Build history of the part. All positions in model axes, mm. Face numbers are marked on the shaded views. A direction names the side the tool comes from. Give positions to 0.01 mm unless a question says otherwise; leave off trailing zeros. Loops run counter-clockwise (first coordinate to the right, second up) from the corner with the lowest first, then second, coordinate; pieces in that order, holes last. Notation, with made-up numbers: M 46,19 L 75,19 A26 cw 75,50 Z; hole C 10.5,63.5 d4. An arc over 180 degrees is marked long. Put each result on its own line as item: value.
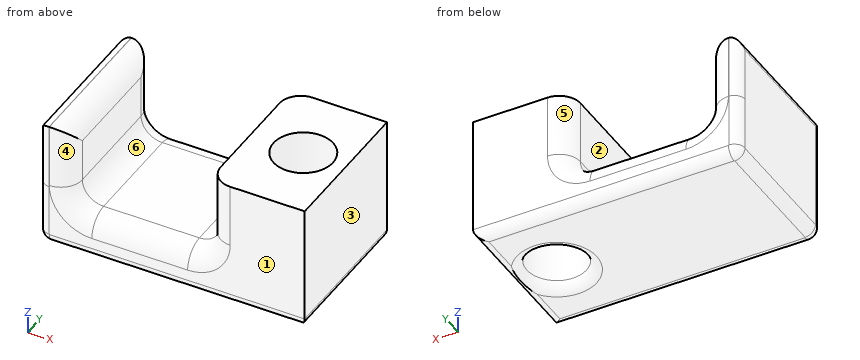
```python
from build123d import *

# Parameters (mm, degrees)
F0_W         = 1.5
F0_H         = 7
F0_W_2       = 6.5
F0_W_3       = 4.5
F0_R         = 1.4
F1_DEPTH     = 2
F2_DEPTH     = 4
F3_F1_R      = 1
F3_F2_R      = 1
F4_T1_DEPTH  = 5.9980686292
F4_T3_DEPTH  = 13.2514489274
F4_T5_DEPTH  = 9.5048292256
F4_T7_DEPTH  = 2.4368940733
F4_T9_DEPTH  = 4.3169803418
F4_T11_DEPTH = 9.509680201
F4_T13_DEPTH = 4.2548401974
F4_T15_DEPTH = 2.4990342177
F4_S19_W     = 0.551502254
F4_S19_H     = 0.5515022539
F4_T20_DEPTH = 0.551502254
F4_S25_W     = 0.551502254
F4_S25_H     = 0.5515022539
F4_T26_DEPTH = 0.551502254


# Not quite as in the source:
# - a fillet or chamfer that OpenCascade refuses, or shapes differently, is made with other operations: its cross-section is extruded or revolved along the edge and cut away or added


with BuildPart() as f1:
    # F0 (on Top) → F1 (new body)
    with BuildSketch(Plane.XY):
        with Locations((-7.4809225276, 0.9873391916)):
            Rectangle(F0_W, F0_H)
        with Locations((-3.4809225276, 0.9873391916)):
            Rectangle(F0_W_2, F0_H)
        with Locations((2.0190774724, 0.9873391916)):
            Rectangle(F0_W_3, F0_H)
        with Locations((2.2690774724, 0.9873391916)):
            Circle(F0_R, mode=Mode.SUBTRACT)
    extrude(amount=-F1_DEPTH)

    # F0 (on Top) → F2 (join)
    with BuildSketch(Plane.XY):
        with Locations((-7.4809225276, 0.9873391916)):
            Rectangle(F0_W, F0_H)
        with Locations((2.0190774724, 0.9873391916)):
            Rectangle(F0_W_3, F0_H)
        with Locations((2.2690774724, 0.9873391916)):
            Circle(F0_R, mode=Mode.SUBTRACT)
    extrude(amount=F2_DEPTH)

    # F3: fillet of radius 1 on 7 edges, made by hand

    # F3_f1
    f3_f1_edges = [f1.edges().sort_by_distance(p)[0] for p in [
        (-0.2309225276, 0.9873391916, 0),
        (-6.7309225276, 0.9873391916, 0),
    ]]
    fillet(f3_f1_edges, radius=F3_F1_R)

    # F3_f2
    f3_f2_edges = [f1.edges().sort_by_distance(p)[0] for p in [
        (-3.4809225276, 4.4873391916, 0),
        (-3.4809225276, -2.5126608084, 0),
        (-6.7309225276, -2.5126608084, 2.5),
        (-6.7309225276, 4.4873391916, 2.5),
        (-6.7309225276, 0.9873391916, 4),
        (-6.4380293088, 4.4873391916, 0.2928932188),
        (-6.4380293088, -2.5126608084, 0.2928932188),
        (-0.5238157464, -2.5126608084, 0.2928932188),
        (-0.5238157464, 4.4873391916, 0.2928932188),
    ]]
    fillet(f3_f2_edges, radius=F3_F2_R)

    # F4: fillet of radius 0.5 on 8 edges, made by hand

    # F4_s2 → F4_t1 (cut)
    with BuildSketch(Plane.XZ.offset(-3.9863735062)):
        with BuildLine():
            ThreePointArc((-8.2313225276, -1.4990343146), (-8.0844759182, -1.8535533906), (-7.7299568422, -2.0004))
            Line((-7.7299568422, -2.0004), (-7.7299568422, -2.0505365685))
            ThreePointArc((-7.7299568422, -2.0505365685), (-7.9804396849, -2.0501365685), (-8.2309225276, -2.0501365685))
            Line((-8.2309225276, -2.0501365685), (-8.2810590962, -2))
            ThreePointArc((-8.2810590962, -2), (-8.2810590962, -1.7495171573), (-8.2814590962, -1.4990343146))
            Line((-8.2814590962, -1.4990343146), (-8.2313225276, -1.4990343146))
        make_face()
    extrude(amount=F4_T1_DEPTH, mode=Mode.SUBTRACT)

    # F4_s4 → F4_t3 (cut)
    with BuildSketch(Plane.YZ.offset(-7.7299568422)):
        with BuildLine():
            ThreePointArc((-2.011695123, -2.0004), (-2.366214199, -1.8535533906), (-2.5130608084, -1.4990343146))
            Line((-2.5130608084, -1.4990343146), (-2.563197377, -1.4990343146))
            ThreePointArc((-2.563197377, -1.4990343146), (-2.562797377, -1.7495171573), (-2.562797377, -2))
            Line((-2.562797377, -2), (-2.5126608084, -2.0501365685))
            ThreePointArc((-2.5126608084, -2.0501365685), (-2.2621779657, -2.0501365685), (-2.011695123, -2.0505365685))
            Line((-2.011695123, -2.0505365685), (-2.011695123, -2.0004))
        make_face()
        with BuildLine():
            ThreePointArc((4.4877391916, -1.4990343146), (4.3408925822, -1.8535533906), (3.9863735062, -2.0004))
            Line((3.9863735062, -2.0004), (3.9863735062, -2.0505365685))
            ThreePointArc((3.9863735062, -2.0505365685), (4.2368563489, -2.0501365685), (4.4873391916, -2.0501365685))
            Line((4.4873391916, -2.0501365685), (4.5374757601, -2))
            ThreePointArc((4.5374757601, -2), (4.5374757601, -1.7495171573), (4.5378757601, -1.4990343146))
            Line((4.5378757601, -1.4990343146), (4.4877391916, -1.4990343146))
        make_face()
    extrude(amount=F4_T3_DEPTH, mode=Mode.SUBTRACT)

    # F4_s6 → F4_t5 (cut)
    with BuildSketch(Plane.XZ.offset(-5.7397538044)):
        with BuildLine():
            ThreePointArc((3.768111787, -2.0004), (4.122630863, -1.8535533906), (4.2694774724, -1.4990343146))
            Line((4.2694774724, -1.4990343146), (4.3196140409, -1.4990343146))
            ThreePointArc((4.3196140409, -1.4990343146), (4.3192140409, -1.7495171573), (4.3192140409, -2))
            Line((4.3192140409, -2), (4.2690774724, -2.0501365685))
            ThreePointArc((4.2690774724, -2.0501365685), (4.0185946297, -2.0501365685), (3.768111787, -2.0505365685))
            Line((3.768111787, -2.0505365685), (3.768111787, -2.0004))
        make_face()
    extrude(amount=F4_T5_DEPTH, mode=Mode.SUBTRACT)

    # F4_s8 → F4_t7 (cut)
    with BuildSketch(Plane.XY.offset(-1.4990343146)):
        with BuildLine():
            ThreePointArc((-8.2313225276, -2.011695123), (-8.0844759182, -2.366214199), (-7.7299568422, -2.5130608084))
            Line((-7.7299568422, -2.5130608084), (-7.7299568422, -2.563197377))
            ThreePointArc((-7.7299568422, -2.563197377), (-7.9804396849, -2.562797377), (-8.2309225276, -2.562797377))
            Line((-8.2309225276, -2.562797377), (-8.2810590962, -2.5126608084))
            ThreePointArc((-8.2810590962, -2.5126608084), (-8.2810590962, -2.2621779657), (-8.2814590962, -2.011695123))
            Line((-8.2814590962, -2.011695123), (-8.2313225276, -2.011695123))
        make_face()
    extrude(amount=F4_T7_DEPTH, mode=Mode.SUBTRACT)

    # F4_s10 → F4_t9 (cut)
    with BuildSketch(Plane.XY.offset(0.9378597587)):
        with BuildLine():
            ThreePointArc((-8.2313225276, -2.0116941886), (-8.0841327357, -2.3665561153), (-7.7289866453, -2.5130589353))
            Line((-7.7289866453, -2.5130589353), (-7.7288896256, -2.56319541))
            ThreePointArc((-7.7288896256, -2.56319541), (-7.7309225276, -2.562797377), (-8.2309225276, -2.562797377))
            Line((-8.2309225276, -2.562797377), (-8.2810590962, -2.5126608084))
            ThreePointArc((-8.2810590962, -2.5126608084), (-8.2810590962, -2.2621774985), (-8.2814590962, -2.0116941886))
            Line((-8.2814590962, -2.0116941886), (-8.2313225276, -2.0116941886))
        make_face()
    extrude(amount=F4_T9_DEPTH, mode=Mode.SUBTRACT)

    # F4_s12 → F4_t11 (cut)
    with BuildSketch(Plane.XZ.offset(-5.7421792921)):
        with BuildLine():
            ThreePointArc((-7.7289866453, 4.0003981269), (-8.0841327357, 3.8538953069), (-8.2313225276, 3.4990333802))
            Line((-8.2313225276, 3.4990333802), (-8.2814590962, 3.4990333802))
            ThreePointArc((-8.2814590962, 3.4990333802), (-8.2810590962, 3.7495166901), (-8.2810590962, 4))
            Line((-8.2810590962, 4), (-8.2309225276, 4.0501365685))
            ThreePointArc((-8.2309225276, 4.0501365685), (-7.7309225276, 4.0501365685), (-7.7288896256, 4.0505346016))
            Line((-7.7288896256, 4.0505346016), (-7.7289866453, 4.0003981269))
        make_face()
    extrude(amount=F4_T11_DEPTH, mode=Mode.SUBTRACT)

    # F4_s14 → F4_t13 (cut)
    with BuildSketch(Plane.XY.offset(0.9999999031)):
        with BuildLine():
            ThreePointArc((-7.7289866453, 4.4877373185), (-8.0841327357, 4.3412344984), (-8.2313225276, 3.9863725718))
            Line((-8.2313225276, 3.9863725718), (-8.2814590962, 3.9863725718))
            ThreePointArc((-8.2814590962, 3.9863725718), (-8.2810590962, 4.2368558817), (-8.2810590962, 4.4873391916))
            Line((-8.2810590962, 4.4873391916), (-8.2309225276, 4.5374757601))
            ThreePointArc((-8.2309225276, 4.5374757601), (-7.7309225276, 4.5374757601), (-7.7288896256, 4.5378737932))
            Line((-7.7288896256, 4.5378737932), (-7.7289866453, 4.4877373185))
        make_face()
    extrude(amount=F4_T13_DEPTH, mode=Mode.SUBTRACT)

    # F4_s16 → F4_t15 (cut)
    with BuildSketch(Plane.XY.offset(-1.4990343146)):
        with BuildLine():
            ThreePointArc((-7.7299568422, 4.4877391916), (-8.0844759182, 4.3408925822), (-8.2313225276, 3.9863735062))
            Line((-8.2313225276, 3.9863735062), (-8.2814590962, 3.9863735062))
            ThreePointArc((-8.2814590962, 3.9863735062), (-8.2810590962, 4.2368563489), (-8.2810590962, 4.4873391916))
            Line((-8.2810590962, 4.4873391916), (-8.2309225276, 4.5374757601))
            ThreePointArc((-8.2309225276, 4.5374757601), (-7.9804396849, 4.5374757601), (-7.7299568422, 4.5378757601))
            Line((-7.7299568422, 4.5378757601), (-7.7299568422, 4.4877391916))
        make_face()
    extrude(amount=F4_T15_DEPTH, mode=Mode.SUBTRACT)


with BuildPart() as f4_tool18:
    # F4_s19 → F4_t20 (new body)
    with BuildSketch(Plane.XZ.offset(-3.9863735062)):
        with Locations((-8.0057079692, -1.7747854416)):
            Rectangle(F4_S19_W, F4_S19_H)
    extrude(amount=-F4_T20_DEPTH)

    # F4_s21 → F4_t22 (revolve, cut)
    with BuildSketch(Plane(origin=(-7.7299568422, 3.9863735062, -1.4990343146), x_dir=(0.7071067812, 0, 0.7071067812), z_dir=(-0.7071067812, 0, 0.7071067812))):
        with BuildLine():
            ThreePointArc((0, -0.5013656854), (0.5013656854, 0), (0, 0.5013656854))
            Line((0, 0.5013656854), (0, -0.5013656854))
        make_face()
    revolve(axis=Axis((-7.7299568422, 3.9863735062, -1.4990343146), (0, 1, 0)), mode=Mode.SUBTRACT)


with BuildPart() as f1_1:
    add(f1.part)

    # F4_t17: cut F4_tool18
    add(f4_tool18.part, mode=Mode.SUBTRACT)


with BuildPart() as f4_tool24:
    # F4_s25 → F4_t26 (new body)
    with BuildSketch(Plane.YZ.offset(-7.7299568422)):
        with Locations((-2.28744625, -1.7747854416)):
            Rectangle(F4_S25_W, F4_S25_H)
    extrude(amount=-F4_T26_DEPTH)

    # F4_s27 → F4_t28 (revolve, cut)
    with BuildSketch(Plane(origin=(-7.7299568422, -2.011695123, -1.4990343146), x_dir=(0, 0.7071067812, 0.7071067812), z_dir=(0, -0.7071067812, 0.7071067812))):
        with BuildLine():
            ThreePointArc((0, -0.5013656854), (0.5013656854, 0), (0, 0.5013656854))
            Line((0, 0.5013656854), (0, -0.5013656854))
        make_face()
    revolve(axis=Axis((-7.7299568422, -2.011695123, -1.4990343146), (-1, 0, 0)), mode=Mode.SUBTRACT)


with BuildPart() as f1_2:
    add(f1_1.part)

    # F4_t23: cut F4_tool24
    add(f4_tool24.part, mode=Mode.SUBTRACT)

    # F4_s29 → F4_t30 (revolve, cut)
    with BuildSketch(Plane.XZ.offset(-0.9873391916)):
        with BuildLine():
            ThreePointArc((4.1700431578, -2.0004), (3.8155240818, -1.8535533906), (3.6686774724, -1.4990343146))
            Line((3.6686774724, -1.4990343146), (3.6185409038, -1.4990343146))
            ThreePointArc((3.6185409038, -1.4990343146), (3.6189409038, -1.7495171573), (3.6189409038, -2))
            Line((3.6189409038, -2), (3.6690774724, -2.0501365685))
            ThreePointArc((3.6690774724, -2.0501365685), (3.9195603151, -2.0501365685), (4.1700431578, -2.0505365685))
            Line((4.1700431578, -2.0505365685), (4.1700431578, -2.0004))
        make_face()
    revolve(axis=Axis((2.2690774724, 0.9873391916, -2), (0, 0, 1)), mode=Mode.SUBTRACT)


solid = f1_2.part
```
Q1. Slice it at A-A (z = 3.75). State how many separate pieces and enclosed holes the cut face has, and give its area (3 significant figures).
Here are the results:
separate pieces: 2
enclosed holes: 1
area: 32.4 mm²
Q2. Mould opens along X. For the marked faces 1, 2 and 3 say: pulls with the +X half, pulls with the -X half, needs draft (parallel to the pull), parting line crosses it, or undercut.
Here are the results:
face 1: needs draft
face 2: undercut
face 3: pulls with the +X half
Q3. Slice it at B-B (x = -3). List the corners of the cut face in (y, z), and give its area (3 significant figures).
Here are the results:
outline: M -2.51,-1.52 A0.5 ccw -2.03,-2 L 4.01,-2 A0.5 ccw 4.49,-1.52 L 4.49,-1 A1 ccw 3.49,0 L -1.51,0 A1 ccw -2.51,-1 Z
area: 13.5 mm²
Q4. Probe line 1 (X direction, y = -0.25, z = 0.5); line 2 (X direction, y = 2.5, z = 1.25); line 3 (X direction, y = 1.25, z = 3). List the from-to ranges inside material, lowest first. Write a range as from..to.
Here are the results:
line 1: -8.23..-6.6, -0.36..1.61, 2.92..4.27
line 2: -8.23..-6.73, -0.23..4.27
line 3: -8.23..-6.73, -0.23..0.89, 3.64..4.27
Q5. Drop a flat-ended pin along its axis: pin 1 Ø1.5 at (x, y) = (-4.5, 1) entering from +Z. Give the stop position or say it passes through.
Here are the results:
pin 1: z = 0
Q6. Tool access for the marked faces 4, 5 and 6: list every direction of +Z, -Z, +X, -X, +Y, -Y with a clear straight run to the whole face (end or side of a thin tool).
Here are the results:
face 4: +Z, -Y
face 5: +Z, +Y
face 6: +Z, +Y, -Y
